```python
from build123d import *

# Parameters (mm, degrees)
SKETCH1_R               = 25
BOSS_EXTRUDE1_DEPTH     = 100
CUT_EXTRUDE1_DEPTH      = 100
CUT_EXTRUDE2_REACH      = 112.567
CUT_EXTRUDE2_END_RADIUS = 25
SKETCH3_W               = 30
SKETCH3_H               = 30
CUT_EXTRUDE3_REACH      = 112.567
CUT_EXTRUDE3_END_RADIUS = 25
SKETCH4_W               = 30
SKETCH4_H               = 30


with BuildPart() as part:
    # Sketch1 → Boss-Extrude1 (new body)
    with BuildSketch(Plane(origin=(0, 0, 0), x_dir=(1, 0, 0), z_dir=(0, 1, 0))):
        with Locations(Location((0, 0, 0), (0, 0, 270))):
            Circle(SKETCH1_R)
    extrude(amount=BOSS_EXTRUDE1_DEPTH)

    # 3DSketch4 → Cut-Extrude1 (cut)
    with BuildSketch(Plane(origin=(-15, 0, -15), x_dir=(0.7071067811865476, 0, 0.7071067811865476), z_dir=(0, 1, 0))):
        Polygon((0, 0), (21.213203436, 21.213203436), (42.426406871, 0), (21.213203436, -21.213203436), align=None)
    extrude(amount=CUT_EXTRUDE1_DEPTH, mode=Mode.SUBTRACT)

    # Cut-Extrude2: up to this cylinder (the profile starts inside it)
    cut_extrude2_end = Plane(origin=(0, 50, 0), z_dir=(0, -1, 0)) * Cylinder(CUT_EXTRUDE2_END_RADIUS, 276.134, mode=Mode.PRIVATE)
    # Sketch3 → Cut-Extrude2 (cut, up to the surface)
    with BuildSketch(Plane.XY.offset(-15), mode=Mode.PRIVATE) as cut_extrude2_sk1:
        with Locations((0, 50)):
            Rectangle(SKETCH3_W, SKETCH3_H)
    cut_extrude2_tool1 = extrude(cut_extrude2_sk1.sketch, amount=-CUT_EXTRUDE2_REACH, mode=Mode.PRIVATE) & cut_extrude2_end
    add(cut_extrude2_tool1.solids().sort_by_distance((0, 50, -15))[0], mode=Mode.SUBTRACT)

    # Cut-Extrude3: up to this cylinder (the profile starts inside it)
    cut_extrude3_end = Plane(origin=(0, 50, 0), z_dir=(0, -1, 0)) * Cylinder(CUT_EXTRUDE3_END_RADIUS, 276.134, mode=Mode.PRIVATE)
    # Sketch4 → Cut-Extrude3 (cut, up to the surface)
    with BuildSketch(Plane(origin=(0, 0, 15), x_dir=(-1, 0, 0), z_dir=(0, 0, -1)), mode=Mode.PRIVATE) as cut_extrude3_sk1:
        with Locations((0, 50)):
            Rectangle(SKETCH4_W, SKETCH4_H)
    cut_extrude3_tool1 = extrude(cut_extrude3_sk1.sketch, amount=-CUT_EXTRUDE3_REACH, mode=Mode.PRIVATE) & cut_extrude3_end
    add(cut_extrude3_tool1.solids().sort_by_distance((0, 50, 15))[0], mode=Mode.SUBTRACT)


solid = part.part
```
Work out the finished part from the listing and answer in its coordinate system (mm). A direction names the side the tool comes from. Coordinates: 2 decimals unless noted, no trailing zeros. Loops run counter-clockwise (first coordinate to the right, second up) from the corner with the lowest first, then second, coordinate; pieces in that order, holes last. Notation, with made-up numbers: (-24, 61.25) - (20, 61.25) arc R25 cw to (20, 76.25) - close; hole circle Ø8 at (7, 17). An arc over 180 degrees is marked (long way). Use a Markdown table: item, result.
Item 1: For faces 1 (the flat face through (0, 65, -19)), 2 (the flat face through (0, 17, -15)), determine the directions among +Z, -Z, +X, -X, +Y, -Y from which every point of the face is accessible in a straight line to the end or side of a thin tool.
Evaluation:
| item | result |
|---|---|
| face 1 | +Z, -Z |
| face 2 | +Y, -Y |
Item 2: Find section D-D, the plane y = 66. Determine the outline of the cut face in (x, z).
Evaluation:
| item | result |
|---|---|
| outline | circle Ø50 at (0, 0); hole (-15, -15) - (15, -15) - (15, 15) - (-15, 15) - close |
Item 3: Given pin 1 Ø5.5 at (y, z) = (46.5, 17) entering from -X; pin 2 Ø1 at (y, z) = (42, -17) entering from +X; pin 3 Ø4 at (y, z) = (42.5, -18) entering from -X; pin 4 Ø5 at (x, z) = (-7, 21) entering from -Y, each flat-ended and moving along its own axis, determine where each tip first touches the part or whether it passes through.
Evaluation:
| item | result |
|---|---|
| pin 1 | stops at x = -20.54 |
| pin 2 | stops at x = 18.78 |
| pin 3 | stops at x = -19.21 |
| pin 4 | stops at y = 0 |
Item 4: Find section B-B, the plane x = 0. Determine the outline of the cut face in (y, z).
Evaluation:
| item | result |
|---|---|
| outline | (0, -25) - (35, -25) - (35, -15) - (0, -15) - close; (0, 15) - (35, 15) - (35, 25) - (0, 25) - close; (65, -25) - (100, -25) - (100, -15) - (65, -15) - close; (65, 15) - (100, 15) - (100, 25) - (65, 25) - close |
Item 5: Consider probe 1 along Y at (x, z) = (-11.5, 19.5); probe 2 along X at (y, z) = (51, 0); probe 3 along X at (y, z) = (7.5, -8). Determine where each line is inside the solid, lowest interval first. Write a range as from..to.
Evaluation:
| item | result |
|---|---|
| probe 1 | y = 0..35, 65..100 |
| probe 2 | x = -25..-15, 15..25 |
| probe 3 | x = -23.69..-15, 15..23.69 |
Item 6: Find section C-C, the plane y = 50.5. Determine the outline of the cut face in (x, z).
Evaluation:
| item | result |
|---|---|
| outline | (-15, -20) - (-15, 20) arc R25 ccw to start; (15, -20) arc R25 ccw to (15, 20) - close |
Item 7: Find section A-A, the plane z = 0. Determine the outline of the cut face in (x, y).
Evaluation:
| item | result |
|---|---|
| outline | (-25, 0) - (-15, 0) - (-15, 100) - (-25, 100) - close; (15, 0) - (25, 0) - (25, 100) - (15, 100) - close |
Item 8: The mould has two halves that part along Y. Classify faces 3 (the flat face through (0, 82, -15)), 4 (the flat face through (0, 100, 16)), 5 (the flat face through (0, 65, 19)), 6 (the flat face through (0, 0, 16)): +Y half, -Y half, draft (parallel to the pull), parting line (faces both ways), or undercut.
Evaluation:
| item | result |
|---|---|
| face 3 | draft |
| face 4 | +Y half |
| face 5 | undercut |
| face 6 | -Y half |
